from build123d import *

# Parameters (mm, degrees)
SKETCH1_W           = 40.64
SKETCH1_H           = 19.05
BOSS_EXTRUDE1_DEPTH = 88.9
SKETCH3_R           = 7.9375
CUT_EXTRUDE1_DEPTH  = 20.05


with BuildPart() as part:
    # Sketch1 → Boss-Extrude1 (new body)
    with BuildSketch(Plane.XY):
        Rectangle(SKETCH1_W, SKETCH1_H)
    extrude(amount=-BOSS_EXTRUDE1_DEPTH)

    # Sketch3 → Cut-Extrude1 (cut, through all)
    with BuildSketch(Plane(origin=(0, 9.525, 0), x_dir=(1, 0, 0), z_dir=(0, 1, 0))):
        with Locations((10.795, 44.45)):
            Circle(SKETCH3_R)
    extrude(amount=-CUT_EXTRUDE1_DEPTH, mode=Mode.SUBTRACT)


solid = part.part
Design review of the part built by this model. Coordinates are the model's own, in mm. Give positions to 0.01 mm unless a question says otherwise; leave off trailing zeros. Order: outer loops, then holes, each group sorted by start corner. A loop starts at its lowest first (then second) coordinate and runs counter-clockwise, first axis right, second up. Notation, with made-up numbers: (63, 53.5) - (71, 53.5) arc R14 ccw to (71, 64.5) - close; hole circle Ø11 at (54, 78). An arc over 180 degrees is marked (long way). Write item = value, one per line. Start each with the question number.
Q1. We need section B-B on x = 17. State the section outline as (y, z) points (3 decimals), plus the area to 3 significant figures.
Q2. We need section A-A on z = -44.45. State the section outline as (x, y) points (1 decimal), plus the area to 3 significant figures.
Q3. Mouldability with a two-part tool opening along Z and no side actions: class faces 1 (the face through (9.074, 0.133, -36.701)), 2 (the face through (0, -9.525, -44)), 3 (the face through (0, 0, -88.9)) as released by +Z, released by -Z, zero draft, split by the parting line, or undercut.
Q4. To check wall thickness, follow L1, parallel to X at y = 0.75, z = -44.45; L2, parallel to Z at x = 10.5, y = 5.25; L3, parallel to Z at x = 18, y = -2. State the ranges of each line that lie inside material, in increasing order. Write a range as from..to.
Working result:
q1.outline = (-9.525, -88.9) - (9.525, -88.9) - (9.525, -49.4) - (-9.525, -49.4) - close; (-9.525, -39.5) - (9.525, -39.5) - (9.525, 0) - (-9.525, 0) - close
q1.area = 1,500 mm²
q2.outline = (-20.3, -9.5) - (2.9, -9.5) - (2.9, 9.5) - (-20.3, 9.5) - close; (18.7, -9.5) - (20.3, -9.5) - (20.3, 9.5) - (18.7, 9.5) - close
q2.area = 472 mm²
q3.face_1 = undercut
q3.face_2 = zero draft
q3.face_3 = released by -Z
q4.L1 = -20.32..2.86, 18.73..20.32
q4.L2 = -88.9..-52.38, -36.52..0
q4.L3 = -88.9..-47.78, -41.12..0
